Source: CAD feature listing. Evaluate the final solid. Frame: model axes, mm. A direction names the side the tool comes from. Round coordinates to 2 decimals unless told otherwise and drop trailing zeros. Order: outer loops, then holes, each group sorted by start corner. A loop starts at its lowest first (then second) coordinate and runs counter-clockwise, first axis right, second up. Notation, with made-up numbers: (38, 35.25) - (75, 35.25) arc R19 ccw to (75, 65.25) - close; hole circle Ø10 at (-26, 52). An arc over 180 degrees is marked (long way). Use one line per item in the form item = value. Start each with the question number.
Q1. Ray query, line 1 (X direction, y = 1.9, z = -66); line 2 (X direction, y = 1.4, z = -45). Return the intervals inside material, ascending. Write a range as [from, to].
Q2. Cut plane C-C, the plane z = -45. Return the cut outline in (x, y), and give its area (3 significant figures).
Q3. Pin query (flat end, axial travel): pin 1 Ø1.5 at (x, z) = (-11, 20.5) entering from +Y; pin 2 Ø5.5 at (x, y) = (-21.5, 7.5) entering from -Z; pin 3 Ø1.5 at (y, z) = (9, 37.5) entering from +X. Return the tip coordinate at first contact, or that it passes through.
Q4. Draft query along Z for faces 5 (the flat face through (-1, 4, -1)), 6 (the flat face through (-64.5, 2, 18)), 7 (the flat face through (-1, 2, 70)). Return one class per face: released by +Z, released by -Z, zero draft, split by the parting line, or undercut.
Q5. Cut plane B-B, the plane x = -50. Return the cut outline in (y, z), and give its area (3 significant figures).
Q6. Set-up query: faces 1 (the flat face through (-35.5, 2, 17)), 2 (the flat face through (40, 8, -65)), 3 (the flat face through (-23, 8, 40)), 4 (the flat face through (30, 8, -65)). Return all of +Z, -Z, +X, -X, +Y, -Y with unobstructed straight access to the full face (end or side cutting, diameter ignored); none if empty.
Q7. Cut plane A-A, the plane x = 5. Return the cut outline in (y, z).
Q8. Cut plane D-D, the plane x = -14. Return the cut outline in (y, z), and give its area (3 significant figures).
from build123d import *

# Parameters (mm, degrees)
SKETCH1_W           = 140
SKETCH1_H           = 140
BOSS_EXTRUDE1_DEPTH = 4
SKETCH2_R           = 14.5
CUT_EXTRUDE1_DEPTH  = 4
SKETCH3_R           = 20
CUT_EXTRUDE2_DEPTH  = 10
SKETCH5_R           = 1.6
CUT_EXTRUDE5_DEPTH  = 10
CUT_EXTRUDE6_DEPTH  = 10
SKETCH8_W           = 5
SKETCH8_H           = 10
SKETCH8_W_2         = 10
SKETCH8_H_2         = 5
BOSS_EXTRUDE2_DEPTH = 14
SKETCH9_R           = 1.5
CUT_EXTRUDE7_DEPTH  = 151.931275752
SKETCH10_R          = 1.5
CUT_EXTRUDE8_DEPTH  = 5
FILLET1_R           = 2.5


with BuildPart() as part:
    # Sketch1 → Boss-Extrude1 (new body)
    with BuildSketch(Plane(origin=(0, 0, 0), x_dir=(1, 0, 0), z_dir=(0, 1, 0))):
        Rectangle(SKETCH1_W, SKETCH1_H)
    extrude(amount=BOSS_EXTRUDE1_DEPTH)

    # Sketch2 → Cut-Extrude1 (cut)
    with BuildSketch(Plane(origin=(0, 4, 0), x_dir=(1, 0, 0), z_dir=(0, 1, 0))):
        with Locations(Location((50, 45, 0), (0, 0, 270))):
            Circle(SKETCH2_R)
        with Locations(Location((20, 45, 0), (0, 0, 270))):
            Circle(SKETCH2_R)
        with Locations(Location((-50, -20, 0), (0, 0, 270))):
            Circle(SKETCH2_R)
        with Locations(Location((-50, -50, 0), (0, 0, 270))):
            Circle(SKETCH2_R)
    extrude(amount=-CUT_EXTRUDE1_DEPTH, mode=Mode.SUBTRACT)

    # Sketch3 → Cut-Extrude2 (cut)
    with BuildSketch(Plane(origin=(0, 4, 0), x_dir=(1, 0, 0), z_dir=(0, 1, 0))):
        with Locations(Location((35, -35, 0), (0, 0, 270))):
            Circle(SKETCH3_R)
    extrude(amount=-CUT_EXTRUDE2_DEPTH, mode=Mode.SUBTRACT)

    # Sketch5 → Cut-Extrude5 (cut)
    with BuildSketch(Plane(origin=(0, 4, 0), x_dir=(1, 0, 0), z_dir=(0, 1, 0))):
        with Locations(Location((-66, 66, 0), (0, 0, 270))):
            Circle(SKETCH5_R)
        with Locations(Location((66, 66, 0), (0, 0, 270))):
            Circle(SKETCH5_R)
        with Locations(Location((66, -66, 0), (0, 0, 270))):
            Circle(SKETCH5_R)
        with Locations(Location((-66, -66, 0), (0, 0, 270))):
            Circle(SKETCH5_R)
    extrude(amount=-CUT_EXTRUDE5_DEPTH, mode=Mode.SUBTRACT)

    # Sketch7 → Cut-Extrude6 (cut)
    with BuildSketch(Plane(origin=(0, 4, 0), x_dir=(1, 0, 0), z_dir=(0, 1, 0))):
        with BuildLine():
            Line((-64.5, -20), (-64.5, -15))
            ThreePointArc((-64.5, -15), (-50, -0.5), (-35.5, -15))
            Line((-35.5, -15), (-35.5, -20))
            ThreePointArc((-35.5, -20), (-50, -34.5), (-64.5, -20))
        make_face()
        with BuildLine():
            Line((20, 30.5), (15, 30.5))
            ThreePointArc((15, 30.5), (0.5, 45), (15, 59.5))
            Line((15, 59.5), (20, 59.5))
            ThreePointArc((20, 59.5), (34.5, 45), (20, 30.5))
        make_face()
    extrude(amount=-CUT_EXTRUDE6_DEPTH, mode=Mode.SUBTRACT)

    # Sketch8 → Boss-Extrude2 (add)
    with BuildSketch(Plane(origin=(0, 4, 0), x_dir=(1, 0, 0), z_dir=(0, 1, 0))):
        with Locations((-22.5, -35)):
            Rectangle(SKETCH8_W, SKETCH8_H)
        with Locations((35, 65)):
            Rectangle(SKETCH8_W_2, SKETCH8_H_2)
    extrude(amount=BOSS_EXTRUDE2_DEPTH)

    # Sketch9 → Cut-Extrude7 (cut, through all)
    with BuildSketch(Plane.XY.offset(-62.5)):
        with Locations((35, 12)):
            Circle(SKETCH9_R)
        with BuildLine():
            Line((30, 12), (30, 22.099022081))
            Line((30, 22.099022081), (40, 22.099022081))
            Line((40, 22.099022081), (40, 12))
            ThreePointArc((40, 12), (35, 17), (30, 12))
        make_face()
    extrude(amount=-CUT_EXTRUDE7_DEPTH, mode=Mode.SUBTRACT)

    # Sketch10 → Cut-Extrude8 (cut)
    with BuildSketch(Plane(origin=(-20, 0, 0), x_dir=(0, 0, -1), z_dir=(1, 0, 0))):
        with Locations((-35, 12)):
            Circle(SKETCH10_R)
        with BuildLine():
            Line((-40, 12), (-40, 23.531098802))
            Line((-40, 23.531098802), (-30, 23.531098802))
            Line((-30, 23.531098802), (-30, 12))
            ThreePointArc((-30, 12), (-35, 17), (-40, 12))
        make_face()
    extrude(amount=-CUT_EXTRUDE8_DEPTH, mode=Mode.SUBTRACT)

    # Fillet1
    fillet1_edges = [part.edges().sort_by_distance(p)[0] for p in [
        (33.5, 12, -67.5),
        (33.5, 12, -62.5),
        (-25, 12, 36.5),
        (-20, 12, 36.5),
    ]]
    fillet(fillet1_edges, radius=FILLET1_R - 0.0001)  # a hair under: the kernel refuses the full size


solid = part.part
Completed:
q1.line_1 = [-70, -67.6], [-64.4, 64.4], [67.6, 70]
q1.line_2 = [-70, 0.5], [34.5, 35.5], [64.5, 70]
q2.outline = (-70, 0) - (0.5, 0) - (0.5, 4) - (-70, 4) - close; (34.5, 0) - (35.5, 0) - (35.5, 4) - (34.5, 4) - close; (64.5, 0) - (70, 0) - (70, 4) - (64.5, 4) - close
q2.area = 308 mm2
q3.pin_1 = 4
q3.pin_2 = 30
q3.pin_3 = -20
q4.face_5 = zero draft
q4.face_6 = undercut
q4.face_7 = released by +Z
q5.outline = (0, -70) - (4, -70) - (4, 0.5) - (0, 0.5) - close; (0, 34.5) - (4, 34.5) - (4, 35.5) - (0, 35.5) - close; (0, 64.5) - (4, 64.5) - (4, 70) - (0, 70) - close
q5.area = 308 mm2
q6.face_1 = +Y, -Y
q6.face_2 = +Z, -Z, +X, +Y
q6.face_3 = +Z, +X, -X, +Y
q6.face_4 = +Z, -Z, -X, +Y
q7.outline = (0, -70) - (4, -70) - (4, -55.5) - (0, -55.5) - close; (0, -34.5) - (4, -34.5) - (4, 70) - (0, 70) - close
q8.outline = (0, -70) - (4, -70) - (4, 70) - (0, 70) - close
q8.area = 560 mm2
